Design review of the part built by this model. Coordinates are the model's own, in mm. Face numbers are marked on the shaded views. A direction names the side the tool comes from. Round coordinates to 2 decimals unless told otherwise and drop trailing zeros. Loops run counter-clockwise (first coordinate to the right, second up) from the corner with the lowest first, then second, coordinate; pieces in that order, holes last. Notation, with made-up numbers: M 31,30 L 89,30 A31 cw 89,62 Z; hole C 38,68 d2. An arc over 180 degrees is marked long. Answer as CSV lines item,"result". Start each with the question number.
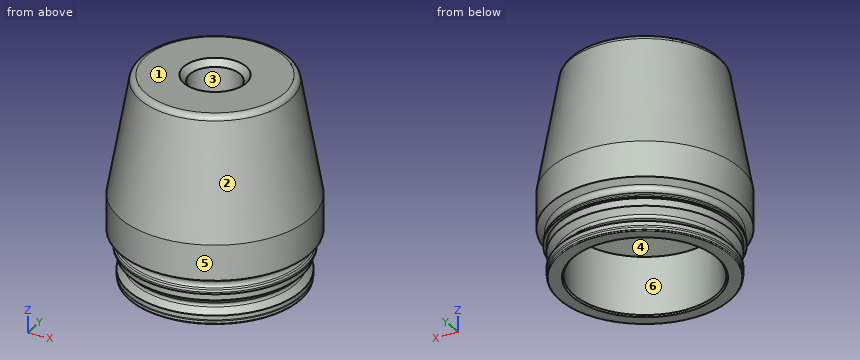
from build123d import *

# Parameters (mm, degrees)
F_5_8_11_TAPPED_HOLE1_D           = 13.49248
F_5_8_11_TAPPED_HOLE1_DEPTH       = 40.1193
F_5_8_11_TAPPED_HOLE1_CSINK_D     = 16.6624
F_5_8_11_TAPPED_HOLE1_CSINK_ANGLE = 90
F_5_8_11_TAPPED_HOLE1_TIP         = 4.053549943
FCH_00_CHAMFER_0_015_SIZE         = 0.381
FILLET1_R                         = 1.5875


with BuildPart() as part:
    # Sketch3 → FBR-00 Basic blank revolve. (revolve)
    with BuildSketch(Plane(origin=(0, 0, 0), x_dir=(0, 0, -1), z_dir=(1, 0, 0)), mode=Mode.PRIVATE) as fbr_00_basic_blank_revolve_sk:
        with BuildLine():
            Line((-45.466, 19.84375), (-45.466, 0))
            Line((-45.466, 0), (-12.115698454, 0))
            Line((-12.115698454, 0), (-7.366, 19.05))
            Line((-7.366, 19.05), (8.509, 19.05))
            Line((8.509, 19.05), (8.509, 22.6695))
            ThreePointArc((8.509, 22.6695), (8.434605122, 22.849105122), (8.255, 22.9235))
            Line((8.255, 22.9235), (7.62, 22.9235))
            Line((7.62, 22.9235), (7.239, 23.0505))
            Line((7.239, 23.0505), (6.096, 23.0505))
            Line((6.096, 23.0505), (4.602815367, 21.557315367))
            ThreePointArc((4.602815367, 21.557315367), (4.064, 21.334130735), (3.525184633, 21.557315367))
            Line((3.525184633, 21.557315367), (2.032, 23.0505))
            Line((2.032, 23.0505), (0, 23.0505))
            Line((0, 23.0505), (0, 23.8125))
            Line((0, 23.8125), (-0.508, 23.8125))
            ThreePointArc((-0.508, 23.8125), (-0.799604775, 23.754496204), (-1.046815367, 23.589315367))
            Line((-1.046815367, 23.589315367), (-1.387974388, 23.248156347))
            ThreePointArc((-1.387974388, 23.248156347), (-2.451768264, 22.887046985), (-3.385852263, 23.511181959))
            Line((-3.385852263, 23.511181959), (-4.476361867, 25.4))
            Line((-4.476361867, 25.4), (-13.95494039, 25.4))
            Line((-13.95494039, 25.4), (-45.466, 19.84375))
        make_face()
    revolve(fbr_00_basic_blank_revolve_sk.sketch.rotate(Axis((0, 0, -27.766671499), (0, 0, 1)), 90), axis=Axis((0, 0, -27.766671499), (0, 0, 1)))

    # 5/8-11 Tapped Hole1
    with Locations(Plane.XY.offset(45.466)):
        with Locations((0, 0)):
            CounterSinkHole(F_5_8_11_TAPPED_HOLE1_D / 2, F_5_8_11_TAPPED_HOLE1_CSINK_D / 2, depth=F_5_8_11_TAPPED_HOLE1_DEPTH, counter_sink_angle=F_5_8_11_TAPPED_HOLE1_CSINK_ANGLE)
            with Locations((0, 0, -(F_5_8_11_TAPPED_HOLE1_DEPTH + F_5_8_11_TAPPED_HOLE1_TIP / 2))):  # 118° drill point
                Cone(0, F_5_8_11_TAPPED_HOLE1_D / 2, F_5_8_11_TAPPED_HOLE1_TIP, mode=Mode.SUBTRACT)

    # FCH-00 Chamfer 0.015
    fch_00_chamfer_0_015_edges = [part.edges().sort_by_distance(p)[0] for p in [
        (19.05, 0, -8.509),
    ]]
    chamfer(fch_00_chamfer_0_015_edges, length=FCH_00_CHAMFER_0_015_SIZE)

    # Fillet1
    fillet1_edges = [part.edges().sort_by_distance(p)[0] for p in [
        (19.84375, 0, 45.466),
    ]]
    fillet(fillet1_edges, radius=FILLET1_R)


solid = part.part
Item 1: Consider section B-B, the plane z = 9. Write out the cut boundary in (x, y).
Item 2: The part is to be moulded in two halves that separate along X. For the marked faces 1, 2, 3 and 4, say which applies: +X half, -X half, draft (parallel to the pull), parting line (faces both ways), or undercut.
Item 3: Tool access review of the marked faces 5 and 6: name each direction out of +Z, -Z, +X, -X, +Y, -Y from which nothing blocks a thin tool from reaching the whole face with its end or side.
Item 4: Consider section A-A, the plane z = 25. Write out the cut boundary in (x, y).
Item 5: To check wall thickness, follow line 1 (Y direction, x = 0, z = 18); line 2 (Y direction, x = -1.5, z = 14.5); line 3 (Y direction, x = 12.5, z = 26). State the ranges of each line that lie inside material, in increasing order.
Item 6: Insertion check: pin 1 Ø2 at (x, z) = (11, 12) entering from +Y; pin 2 Ø4 at (y, z) = (-7, 1) entering from -X; pin 3 Ø12 at (x, z) = (-20, 30.5) entering from +Y. Each pin has a flat end and moves straight along its axis. Give the tip position at first contact, or say it passes through.
Found:
1,outline,"C 0,0 d50.8; hole C 0,0 d24.99"
2,face 1,"draft"
2,face 2,"parting line"
2,face 3,"undercut"
2,face 4,"undercut"
3,face 5,"+Z, -Z"
3,face 6,"-Z"
4,outline,"C 0,0 d46.9; hole C 0,0 d13.49"
5,line 1,"y = -24.69 to -6.75, 6.75 to 24.69"
5,line 2,"y = -25.26 to -6.58, 6.58 to 25.26"
5,line 3,"y = -19.63 to 19.63"
6,pin 1,"stops at y = 23.35"
6,pin 2,"stops at x = -23.27"
6,pin 3,"stops at y = 17.78"
